Input: part model. Units: mm. Frame: model coordinates. A direction names the side the tool comes from. Coordinates: 2 decimals unless noted, no trailing zeros. Loops run counter-clockwise (first coordinate to the right, second up) from the corner with the lowest first, then second, coordinate; pieces in that order, holes last.
(1) Line query: L1, parallel to Z at x = 65.3, y = 0; L2, parallel to Z at x = 70.15, y = -12.5 (3 decimals); L3, parallel to X at y = -15, z = 159. Output: solid intervals per line, ascending.
(2) Section A-A, the plane z = 20. Return loops of the section in (x, y), then the cut area to 3 significant figures.
(3) Section B-B, the plane z = 190.5. Return loops of the section in (x, y), then the cut area to 3 significant figures.
(4) Set-up query: faces 4 (the face through (65, 0, 29.8)), 5 (the face through (62, -10.5, 152)), 6 (the face through (67.9, 12, 10)). Return all of +Z, -Z, +X, -X, +Y, -Y with unobstructed straight access to the full face (end or side cutting, diameter ignored); none if empty.
(5) Mould query, pull axis Y, two halves, no side actions, for faces 1 (the face through (55.454, 21.7, 205.28)), 2 (the face through (71.9, 0, 114)), 3 (the face through (67.9, 0, 205)). Classes: released by +Y, released by -Y, zero draft, split by the parting line, or undercut.
(6) Contact query for flat-ended pins moving along their axis: P1, Ø4, axis at y = 0, z = 205, coming from the -X side; P2, Ø12, axis at x = 55, y = -4.5, coming from the -Z side; P3, Ø9, axis at x = 62.25, z = 144.5, coming from the +Y side. Output: stop coordinate, or through.
```python
from build123d import *

# Parameters (mm, degrees)
SKETCH022_R         = 7.5
SKETCH022_R_2       = 1.125
PAD002_DEPTH        = 9.4
HOLE007_D           = 4
HOLE007_CBORE_D     = 7.2
HOLE007_CBORE_DEPTH = 4.2
POCKET005_DEPTH     = 5
PAD003_DEPTH        = 40
POCKET006_DEPTH     = 12.5
SKETCH030_W         = 35
SKETCH030_H         = 88.4
POCKET008_DEPTH     = 5.3
POCKET009_DEPTH     = 8
SKETCH039_W         = 21
SKETCH039_H         = 31.5
POCKET013_DEPTH     = 5
PAD006_DEPTH        = 7
HOLE008_D           = 3.3
HOLE008_DEPTH       = 20
HOLE008_CBORE_D     = 5.7
HOLE008_CBORE_DEPTH = 4.5
HOLE008_TIPS_R      = 1.65
HOLE009_D           = 3.2
HOLE009_DEPTH       = 11
HOLE009_CBORE_D     = 7.2
HOLE009_CBORE_DEPTH = 4.2
SKETCH042_R         = 4.841694
SKETCH042_R_2       = 4.912123
SKETCH042_R_3       = 5.957845
PAD007_DEPTH        = 0.2


with BuildPart() as part:
    # Sketch022 → Pad002 (new body)
    with BuildSketch(Plane.YZ.offset(62.5)):
        Polygon((-17.5, 225), (-17.5, 4.7), (-12.3, 4.7), (-12.3, 0), (12.3, 0), (12.3, 4.7), (17.5, 4.7), (17.5, 225), align=None)
        with Locations((0, 20)):
            Circle(SKETCH022_R, mode=Mode.SUBTRACT)
        with Locations((-12.5, 114.2)):
            Circle(SKETCH022_R_2, mode=Mode.SUBTRACT)
        with Locations((12.5, 114.2)):
            Circle(SKETCH022_R_2, mode=Mode.SUBTRACT)
        with Locations((-12.5, 38.45)):
            Circle(SKETCH022_R_2, mode=Mode.SUBTRACT)
        with Locations((12.5, 38.45)):
            Circle(SKETCH022_R_2, mode=Mode.SUBTRACT)
        with BuildLine():
            ThreePointArc((-8, 34.7), (-10.3, 32.4), (-8, 30.1))
            Line((-8, 30.1), (8, 30.1))
            ThreePointArc((8, 30.1), (10.3, 32.4), (8, 34.7))
            Line((-8, 34.7), (8, 34.7))
        make_face(mode=Mode.SUBTRACT)
    extrude(amount=PAD002_DEPTH)

    # Hole007 (through all)
    with Locations(Plane.YZ.offset(71.9)):
        with Locations((-12.5, 10), (12.5, 10)):
            CounterBoreHole(HOLE007_D / 2, HOLE007_CBORE_D / 2, HOLE007_CBORE_DEPTH)

    # Sketch026 → Pocket005 (cut)
    with BuildSketch(Plane.YZ.offset(69.9)):
        with BuildLine():
            ThreePointArc((-10.8, 34.75), (-13.15, 32.4), (-10.8, 30.05))
            Line((-10.8, 30.05), (10.8, 30.05))
            ThreePointArc((10.8, 30.05), (13.15, 32.4), (10.8, 34.75))
            Line((-10.8, 34.75), (10.8, 34.75))
        make_face()
    extrude(amount=-POCKET005_DEPTH, mode=Mode.SUBTRACT)

    # Sketch027 → Pad003 (join)
    with BuildSketch(Plane.XY.offset(225)):
        with BuildLine():
            ThreePointArc((43.918246, -18.095238), (47.5, 0), (43.918246, 18.095238))
            ThreePointArc((51.101403, 24.294818), (45.274345, 23.785172), (43.918246, 18.095238))
            Line((51.101403, 24.294818), (62.5, 17.5))
            Line((62.5, 17.5), (62.5, -17.5))
            Line((62.5, -17.5), (51.101403, -24.294818))
            ThreePointArc((43.918246, -18.095238), (45.274345, -23.785172), (51.101403, -24.294818))
        make_face()
    extrude(amount=-PAD003_DEPTH)

    # Sketch028 → Pocket006 (cut, symmetric)
    with BuildSketch(Plane.XY.offset(205)):
        with BuildLine():
            ThreePointArc((51.961524, -30), (60, 0), (51.961524, 30))
            Line((51.961524, 30), (62.5, 30))
            Line((62.5, 30), (62.5, -30))
            Line((62.5, -30), (51.961524, -30))
        make_face()
    extrude(amount=POCKET006_DEPTH, both=True, mode=Mode.SUBTRACT)

    # Sketch030 → Pocket008 (cut)
    with BuildSketch(Plane.YZ.offset(62.5)):
        with Locations((0, 74)):
            Rectangle(SKETCH030_W, SKETCH030_H)
    extrude(amount=POCKET008_DEPTH, mode=Mode.SUBTRACT)

    # Sketch031 → Pocket009 (cut)
    with BuildSketch(Plane.YZ.offset(62.5)):
        with BuildLine():
            ThreePointArc((13.845935, 107.277863), (12.783162, 108.340636), (11.720389, 107.277863))
            Line((11.720389, 107.277863), (11.720389, 84.030329))
            ThreePointArc((11.720389, 84.030329), (12.783162, 82.967556), (13.845935, 84.030329))
            Line((13.845935, 107.277863), (13.845935, 84.030329))
        make_face()
        with BuildLine():
            ThreePointArc((-13.393928, 109.875952), (-14.456701, 108.813179), (-13.393928, 107.750406))
            Line((-13.393928, 107.750406), (6.990506, 107.750406))
            ThreePointArc((6.990506, 107.750406), (8.053279, 108.813179), (6.990506, 109.875952))
            Line((-13.393928, 109.875952), (6.990506, 109.875952))
        make_face()
        with BuildLine():
            ThreePointArc((-13.495995, 94.718798), (-14.558768, 93.656025), (-13.495995, 92.593252))
            Line((-13.495995, 92.593252), (6.969508, 92.593252))
            ThreePointArc((6.969508, 92.593252), (8.032281, 93.656025), (6.969508, 94.718798))
            Line((-13.495995, 94.718798), (6.969508, 94.718798))
        make_face()
    extrude(amount=POCKET009_DEPTH, mode=Mode.SUBTRACT)

    # Sketch039 → Pocket013 (cut)
    with BuildSketch(Plane.YZ.offset(62.5)):
        with Locations((0, 152)):
            Rectangle(SKETCH039_W, SKETCH039_H)
    extrude(amount=POCKET013_DEPTH, mode=Mode.SUBTRACT)

    # Sketch040 → Pad006 (join)
    with BuildSketch(Plane.XZ.offset(10.5)):
        with BuildLine():
            Line((62.5, 167.75), (60, 167.75))
            ThreePointArc((60, 167.75), (58.232233, 167.017767), (57.5, 165.25))
            Line((57.5, 165.25), (57.5, 138.75))
            ThreePointArc((57.5, 138.75), (58.232233, 136.982233), (60, 136.25))
            Line((60, 136.25), (62.5, 136.25))
            Line((62.5, 136.25), (62.5, 167.75))
        make_face()
    extrude(amount=PAD006_DEPTH)

    # Hole008
    with Locations(Plane.XZ.offset(17.5)):
        with Locations((62.25, 159.5), (62.25, 144.5)):
            CounterBoreHole(HOLE008_D / 2, HOLE008_CBORE_D / 2, HOLE008_CBORE_DEPTH, depth=HOLE008_DEPTH)

    # Hole008 tips → Hole008 tip 1 section 0
    with BuildSketch(Plane.XZ.offset(-2.5), mode=Mode.PRIVATE) as hole008_tip_1_s0:
        with Locations((62.25, 159.5)):
            Circle(HOLE008_TIPS_R)
    loft([hole008_tip_1_s0.sketch, Vertex(62.25, 3.49142, 159.5)], mode=Mode.SUBTRACT)

    # Hole008 tips → Hole008 tip 2 section 0
    with BuildSketch(Plane.XZ.offset(-2.5), mode=Mode.PRIVATE) as hole008_tip_2_s0:
        with Locations((62.25, 144.5)):
            Circle(HOLE008_TIPS_R)
    loft([hole008_tip_2_s0.sketch, Vertex(62.25, 3.49142, 144.5)], mode=Mode.SUBTRACT)

    # Hole009
    with Locations(Plane.YZ.offset(71.9)):
        with Locations((0, 205)):
            CounterBoreHole(HOLE009_D / 2, HOLE009_CBORE_D / 2, HOLE009_CBORE_DEPTH, depth=HOLE009_DEPTH)

    # Sketch042 → Pad007 (join)
    with BuildSketch(Plane.YZ.offset(67.7)):
        with Locations((-12.26765, 9.945303)):
            Circle(SKETCH042_R)
        with Locations((12.134341, 9.945303)):
            Circle(SKETCH042_R_2)
        with Locations((0, 205)):
            Circle(SKETCH042_R_3)
    extrude(amount=PAD007_DEPTH)


solid = part.part
```
Report:
1. L1: z = 0 to 12.5, 27.5 to 29.8, 118.2 to 136.25, 167.75 to 203.4, 206.6 to 225
1. L2: z = 4.7 to 6.4, 13.6 to 37.325, 39.575 to 92.593, 94.719 to 107.75, 109.876 to 113.075, 115.325 to 225
1. L3: x = 57.5 to 59.44, 65.06 to 71.9
2. outline: (62.5, -17.5) - (71.9, -17.5) - (71.9, -7.5) - (62.5, -7.5) - close; (62.5, 7.5) - (71.9, 7.5) - (71.9, 17.5) - (62.5, 17.5) - close
2. area: 188 mm2
3. outline: (43.92, -18.1) arc R5 ccw to (51.1, -24.29) - (62.5, -17.5) - (71.9, -17.5) - (71.9, 17.5) - (62.5, 17.5) - (51.1, 24.29) arc R5 ccw to (43.92, 18.1) arc R47.5 cw to start
3. area: 1,070 mm2
4. face 4: -X, +Y, -Y
4. face 5: -X
4. face 6: +X
5. face 1: released by +Y
5. face 2: zero draft
5. face 3: undercut
6. P1: stops at x = 47.46
6. P2: stops at z = 185
6. P3: stops at y = 17.5
